```python
from build123d import *

# Parameters (mm, degrees)
F0_W     = 47
F0_H     = 22.9
F1_DEPTH = 17.25
F0_R     = 2.75
F2_DEPTH = 6.95
F0_R_2   = 1.7
F3_DEPTH = 14
F0_R_3   = 2.02
F4_DEPTH = 4.4


with BuildPart() as f1:
    # F0 (on Top) → F1 (new body)
    with BuildSketch(Plane.XY):
        Rectangle(F0_W, F0_H)
        with BuildLine():
            Line((-14.4, 8.825), (-14.4, 9.95))
            Line((-14.4, 9.95), (14.4, 9.95))
            Line((14.4, 9.95), (14.4, -1.075))
            Line((14.4, -1.075), (18, -1.075))
            ThreePointArc((18, -1.075), (21.875, -4.95), (18, -8.825))
            Line((18, -8.825), (14.4, -8.825))
            Line((14.4, -8.825), (14.4, -9.95))
            Line((14.4, -9.95), (-14.4, -9.95))
            Line((-14.4, -9.95), (-14.4, 1.075))
            Line((-14.4, 1.075), (-18, 1.075))
            ThreePointArc((-18, 1.075), (-21.875, 4.95), (-18, 8.825))
            Line((-18, 8.825), (-14.4, 8.825))
        make_face(mode=Mode.SUBTRACT)
    extrude(amount=F1_DEPTH)

    # F0 (on Top) → F2 (join)
    with BuildSketch(Plane.XY):
        Polygon((14.4, 9.95), (-14.4, 9.95), (-14.4, 8.825), (-14.4, 1.075), (-14.4, -9.95), (14.4, -9.95), (14.4, -8.825), (14.4, -1.075), align=None)
        with Locations((-6.35, 3.45)):
            Circle(F0_R, mode=Mode.SUBTRACT)
        with Locations((6.35, 3.45)):
            Circle(F0_R, mode=Mode.SUBTRACT)
    extrude(amount=F2_DEPTH)

    # F0 (on Top) → F3 (join)
    with BuildSketch(Plane.XY):
        with BuildLine():
            Line((18, -1.075), (14.4, -1.075))
            Line((14.4, -1.075), (14.4, -8.825))
            Line((14.4, -8.825), (18, -8.825))
            ThreePointArc((18, -8.825), (21.875, -4.95), (18, -1.075))
        make_face()
        with Locations((18, -4.95)):
            Circle(F0_R_2, mode=Mode.SUBTRACT)
        with BuildLine():
            Line((-14.4, 1.075), (-14.4, 8.825))
            Line((-14.4, 8.825), (-18, 8.825))
            ThreePointArc((-18, 8.825), (-21.875, 4.95), (-18, 1.075))
            Line((-18, 1.075), (-14.4, 1.075))
        make_face()
        with Locations((-18, 4.95)):
            Circle(F0_R_2, mode=Mode.SUBTRACT)
    extrude(amount=F3_DEPTH)

    # F0 (on Top) → F4 (join)
    with BuildSketch(Plane.XY):
        with Locations((-6.35, 3.45)):
            Circle(F0_R)
        with Locations((-6.35, 3.45)):
            Circle(F0_R_3, mode=Mode.SUBTRACT)
        with Locations((6.35, 3.45)):
            Circle(F0_R)
        with Locations((6.35, 3.45)):
            Circle(F0_R_3, mode=Mode.SUBTRACT)
    extrude(amount=F4_DEPTH)


solid = f1.part
```
For this review, take the finished solid that the model builds, in its own axes (mm). A direction names the side the tool comes from. Give positions to 0.01 mm unless a question says otherwise; leave off trailing zeros. Write each loop counter-clockwise with the first axis right and the second up, starting at its lowest first coordinate (ties: lowest second). Pieces come first, ordered by that corner, then holes.
Item 1: The part is to be moulded in two halves that separate along Y. For faces 1 (the face through (0, 11.45, 9)), 2 (the face through (-23.5, 0, 9)), 3 (the face through (8.216, 2.676, 2.169)), say which applies: +Y half, -Y half, draft (parallel to the pull), parting line (faces both ways), or undercut.
Item 2: Take a section at D-D (z = 10). Give the boundary of the cut face in (x, y).
Item 3: Wall thickness on probe 1 along Y at (x, z) = (-3.5, 14); probe 2 along Y at (x, z) = (6.35, 1.9); probe 3 along X at (y, z) = (-0.25, 9): over which ranges is each line inside the solid? List them lowest first.
Item 4: Machinability: for faces 4 (the face through (16, -8.825, 16)), 5 (the face through (-17.086, 6.383, 6.902)), which of the approach directions +Z, -Z, +X, -X, +Y, -Y give a long, thin tool a straight path to every point of the face, cutting with its end or side? Answer none if there is none.
Item 5: Insertion check: P1, Ø6.5, axis at x = 6.35, y = 3.45, coming from the +Z side. The pin has a flat end and moves straight along its axis. Give the tip position at first contact, or say it passes through.
Item 6: Take a section at C-C (z = 3.5). Give the boundary of the cut face in (x, y).
Item 7: Take a section at B-B (x = 6.35). Give the boundary of the cut face in (y, z).
Item 8: Take a section at A-A (y = -4.95). Give the boundary of the cut face in (x, z) (3 decimals), and give its area (3 significant figures).
Established:
1. face 1: +Y half
1. face 2: draft
1. face 3: undercut
2. outline: (-23.5, -11.45) - (23.5, -11.45) - (23.5, 11.45) - (-23.5, 11.45) - close; hole circle Ø3.4 at (-18, 4.95); hole (-14.4, -9.95) - (14.4, -9.95) - (14.4, 9.95) - (-14.4, 9.95) - close; hole circle Ø3.4 at (18, -4.95)
3. probe 1: y = -11.45 to -9.95, 9.95 to 11.45
3. probe 2: y = -11.45 to 1.43, 5.47 to 11.45
3. probe 3: x = -23.5 to -14.4, 14.4 to 23.5
4. face 4: +Z
4. face 5: +Z, -Z
5. P1: stops at z = 6.95
6. outline: (-23.5, -11.45) - (23.5, -11.45) - (23.5, 11.45) - (-23.5, 11.45) - close; hole circle Ø3.4 at (-18, 4.95); hole circle Ø4.04 at (-6.35, 3.45); hole circle Ø4.04 at (6.35, 3.45); hole circle Ø3.4 at (18, -4.95)
7. outline: (-11.45, 0) - (1.43, 0) - (1.43, 4.4) - (0.7, 4.4) - (0.7, 6.95) - (-9.95, 6.95) - (-9.95, 17.25) - (-11.45, 17.25) - close; (5.47, 0) - (11.45, 0) - (11.45, 17.25) - (9.95, 17.25) - (9.95, 6.95) - (6.2, 6.95) - (6.2, 4.4) - (5.47, 4.4) - close
8. outline: (-23.5, 0) - (16.3, 0) - (16.3, 14) - (14.4, 14) - (14.4, 6.95) - (-14.4, 6.95) - (-14.4, 17.25) - (-23.5, 17.25) - close; (19.7, 0) - (23.5, 0) - (23.5, 17.25) - (21.875, 17.25) - (21.875, 14) - (19.7, 14) - close
8. area: 442 mm2
